```python
from build123d import *

# Parameters (mm, degrees)
BOSS_EXTRUDE1_DEPTH  = 25.4
CUT_SWEEP1_START     = 4.000000128
CUT_SWEEP1_OUTLINE_R = 5.750000057
CUT_SWEEP1_DEPTH     = 33.044274766
CUT_SWEEP2_PROFILE_R = 3.499999985
CUT_EXTRUDE1_DEPTH   = 88.74529292


# Read off the part's stored shape, not the designer's step: Cut-Sweep1
with BuildPart() as part:
    # Sketch1 → Boss-Extrude1 (new, symmetric)
    with BuildSketch(Plane(origin=(0, 0, 0), x_dir=(1, 0, 0), z_dir=(0, 1, 0))):
        Polygon((-37.260478906, -42.917333336), (-40.088906121, -40.088906121), (-45.477059794, -45.477059794), (-28.736819587, -62.2173), (-17.960512242, -62.2173), align=None)
        with BuildLine():
            ThreePointArc((35.014018616, -35.014018616), (0, -49.5173), (-35.014018616, -35.014018616))
            Line((-35.014018616, -35.014018616), (-40.088906121, -40.088906121))
            Line((-40.088906121, -40.088906121), (-37.260478906, -42.917333336))
            Line((-37.260478906, -42.917333336), (-17.960512242, -62.2173))
            Line((-17.960512242, -62.2173), (0, -62.2173))
            Line((0, -62.2173), (28.736819587, -62.2173))
            Line((28.736819587, -62.2173), (45.477059794, -45.477059794))
            Line((45.477059794, -45.477059794), (35.014018616, -35.014018616))
        make_face()
        with BuildLine():
            Line((42.917333336, 37.260478906), (40.088906121, 40.088906121))
            Line((40.088906121, 40.088906121), (35.014018616, 35.014018616))
            ThreePointArc((35.014018616, 35.014018616), (45.748019975, 18.949450325), (49.5173, 0))
            ThreePointArc((49.5173, 0), (45.748019975, -18.949450325), (35.014018616, -35.014018616))
            Line((35.014018616, -35.014018616), (45.477059794, -45.477059794))
            Line((45.477059794, -45.477059794), (62.2173, -28.736819587))
            Line((62.2173, -28.736819587), (62.2173, 0))
            Line((62.2173, 0), (62.2173, 17.960512242))
            Line((62.2173, 17.960512242), (42.917333336, 37.260478906))
        make_face()
        Polygon((62.2173, 28.736819587), (45.477059794, 45.477059794), (40.088906121, 40.088906121), (42.917333336, 37.260478906), (62.2173, 17.960512242), align=None)
    extrude(amount=BOSS_EXTRUDE1_DEPTH, both=True)

    # Cut-Sweep1 outline → Cut-Sweep1 (cut)
    with BuildSketch(Plane(origin=(0, 0, 0), x_dir=(0.7071067811865471, 0, -0.707106781186548), z_dir=(0.707106781186548, 0, 0.707106781186547)).offset(CUT_SWEEP1_START)):
        with Locations((-56.694274737, 0)):
            Circle(CUT_SWEEP1_OUTLINE_R)
    extrude(amount=CUT_SWEEP1_DEPTH, mode=Mode.SUBTRACT)

    # Cut-Sweep2: sweep along a path in Sketch44
    with BuildLine(Plane(origin=(0, 0, 0), x_dir=(1, 0, 0), z_dir=(0, 1, 0))) as cut_sweep2_path:
        Line((-40.088906121, -40.088906121), (-37.260478906, -42.917333336))
    # Cut-Sweep2 profile (on start of the path) → Cut-Sweep2 (sweep, cut)
    with BuildSketch(Plane(origin=(-40.088906121, 0, 40.088906121), x_dir=(0.7071067811865493, 0, -0.7071067811865458), z_dir=(0.7071067811865458, 0, 0.7071067811865493))):
        Circle(CUT_SWEEP2_PROFILE_R)
    cut_sweep2 = sweep(path=cut_sweep2_path.line, mode=Mode.SUBTRACT)

    # Mirror1: Cut-Sweep2 across plane
    add(cut_sweep2.mirror(Plane(origin=(0, 0, 0), x_dir=(0.7071067811865477, 0, 0.7071067811865474), z_dir=(-0.7071067811865476, 0, 0.7071067811865476))), mode=Mode.SUBTRACT)

    # Sketch53 → Cut-Extrude1 (cut, through all)
    with BuildSketch(Plane(origin=(2.828427215, 0, 2.828427215), x_dir=(-0.7071067811865427, 0, 0.7071067811865525), z_dir=(-0.7071067811865525, 0, -0.7071067811865427))):
        Polygon((-62.756452611, 0), (-59.725363674, -5.250000041), (-53.6631858, -5.250000041), (-50.632096863, 0), (-53.6631858, 5.250000041), (-59.725363674, 5.250000041), align=None)
    extrude(amount=-CUT_EXTRUDE1_DEPTH, mode=Mode.SUBTRACT)


solid = part.part
```
Design review of the part built by this model. Coordinates are the model's own, in mm. A direction names the side the tool comes from. Coordinates: 2 decimals unless noted, no trailing zeros. Order: outer loops, then holes, each group sorted by start corner. A loop starts at its lowest first (then second) coordinate and runs counter-clockwise, first axis right, second up. Notation, with made-up numbers: (61.25, 8.25) -> (88.25, 8.25) arc R10 ccw to (88.25, 22.25) -> close; hole circle Ø9 at (14, 60). An arc over 180 degrees is marked (long way). One line per item, written item: value. Start each with the question number.
Q1. Take a section at C-C, the plane z = 0. State the section outline as (x, y) points.
Q2. Take a section at D-D, the plane x = 9.5. State the section outline as (y, z) points, then the cut area to 3 significant figures.
Q3. Take a section at B-B, the plane x = 51. State the section outline as (y, z) points.
Q4. Insertion check: pin 1 Ø5 at (y, z) = (13.5, 23.5) entering from -X. The pin has a flat end and moves straight along its axis. Give the tip position at first contact, or say it passes through.
Q5. Tool access review of faces 4 (the flat face through (54, -5.25, -27)), 5 (the flat face through (62.217, 0, 0)): name each direction out of +Z, -Z, +X, -X, +Y, -Y from which nothing blocks a thin tool from reaching the whole face with its end or side.
Q6. Mouldability with a two-part tool opening along X and no side actions: class faces 1 (the flat face through (36, -25.4, 36)), 2 (the flat face through (51.32, 2.59, -22.4)), 3 (the flat face through (43, 0, -43)) as pulls with the +X half, pulls with the -X half, needs draft (parallel to the pull), parting line crosses it, or undercut.
Q7. For probe 1 along X at (y, z) = (-6, 1.5); probe 2 along X at (y, z) = (18, 36); probe 3 along Z at (x, y) = (15, -5.5), list the stretches that pass through material, from the lowest coordinate up.
Values follow:
1. outline: (49.52, -25.4) -> (62.22, -25.4) -> (62.22, 25.4) -> (49.52, 25.4) -> close
2. outline: (-25.4, 48.6) -> (25.4, 48.6) -> (25.4, 62.22) -> (-25.4, 62.22) -> close
2. area: 692 mm2
3. outline: (-25.4, -39.95) -> (25.4, -39.95) -> (25.4, 39.95) -> (-25.4, 39.95) -> close; hole (-5.25, -33.46) -> (0, -37.75) -> (5.25, -33.46) -> (5.25, -24.89) -> (0, -20.6) -> (-5.25, -24.89) -> close
4. pin 1: stops at x = 42.14
5. face 4: none
5. face 5: +Z, -Z, +X, +Y, -Y
6. face 1: needs draft
6. face 2: undercut
6. face 3: pulls with the -X half
7. probe 1: x = 49.49 to 62.22
7. probe 2: x = -36 to -34, 34 to 54.95
7. probe 3: z = 47.19 to 62.22
